from build123d import *

# Parameters (mm, degrees)
BOSS_EXTRUDE1_DEPTH = 25
SKETCH2_R           = 1.75
CUT_EXTRUDE1_DEPTH  = 40.67366885


with BuildPart() as part:
    # Sketch1 → Boss-Extrude1 (new, symmetric)
    with BuildSketch(Plane(origin=(0, 0, 0), x_dir=(0, 0, -1), z_dir=(1, 0, 0))):
        with BuildLine():
            Line((-10, 15), (-10, 0))
            Line((-10, 0), (-18, 0))
            Line((-18, 0), (-18, 1.5))
            Line((-18, 1.5), (-11.5, 1.5))
            Line((-11.5, 1.5), (-11.5, 15))
            ThreePointArc((-11.5, 15), (0, 26.5), (11.5, 15))
            Line((11.5, 15), (11.5, 1.5))
            Line((11.5, 1.5), (18, 1.5))
            Line((18, 1.5), (18, 0))
            Line((18, 0), (10, 0))
            Line((10, 0), (10, 15))
            ThreePointArc((10, 15), (0, 25), (-10, 15))
        make_face()
    extrude(amount=BOSS_EXTRUDE1_DEPTH, both=True)

    # Sketch2 → Cut-Extrude1 (cut, through all)
    with BuildSketch(Plane(origin=(0, 1.5, 0), x_dir=(1, 0, 0), z_dir=(0, 1, 0))):
        with Locations(Location((-15, 14.75, 0), (0, 0, 270))):
            Circle(SKETCH2_R)
        with Locations(Location((-15, -14.75, 0), (0, 0, 270))):
            Circle(SKETCH2_R)
    cut_extrude1 = extrude(amount=-CUT_EXTRUDE1_DEPTH, mode=Mode.SUBTRACT)

    # Mirror1: Cut-Extrude1 across plane
    add(cut_extrude1.mirror(Plane(origin=(0, 0, 0), x_dir=(0, 0, 1), z_dir=(1, 0, 0))), mode=Mode.SUBTRACT)


solid = part.part
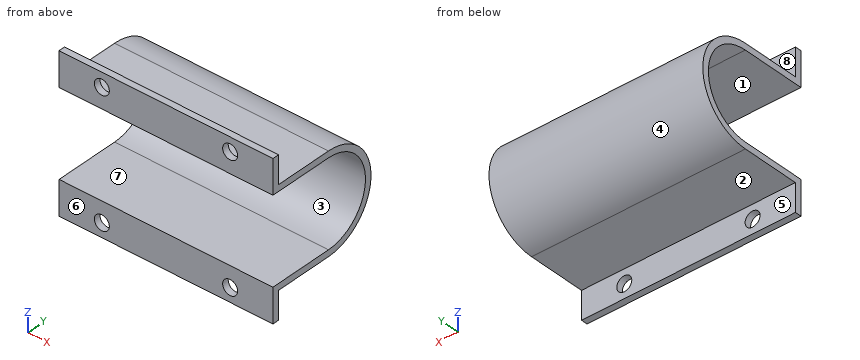
For this review, take the finished solid that the model builds, in its own axes (mm). Face numbers are marked on the shaded views. A direction names the side the tool comes from. Round coordinates to 2 decimals unless told otherwise and drop trailing zeros. Write each loop counter-clockwise with the first axis right and the second up, starting at its lowest first coordinate (ties: lowest second). Pieces come first, ordered by that corner, then holes. Notation, with made-up numbers: M 58.25,80.25 L 105.25,80.25 A9 cw 105.25,88.25 Z; hole C 76,63.25 d10. An arc over 180 degrees is marked long. Write item = value, one per line. Start each with the question number.
(1) For the marked faces 5, 6, 7 and 8, list the 3-axis set-ups (+Z, -Z, +X, -X, +Y, -Y) from which the entire face can be reached by the end or side of a thin tool; tool diameter is ignored.
(2) We need section B-B (x = 15). Give the boundary of the cut face in (y, z), then the cut area to 3 significant figures.
(3) Clearance check with flat-ended pins moving along their axes: pin 1 Ø10 at (x, y) = (18, 11) entering from +Z; pin 2 Ø6 at (x, y) = (11.5, 8.5) entering from -Z; pin 3 Ø10 at (x, y) = (-2.5, 22) entering from -Z; pin 4 Ø2 at (x, z) = (15, -14.75) entering from -Y. State where each tip first meets the part, or that it passes through.
(4) We need section C-C (y = 7.5). Give the boundary of the cut face in (x, z), then the cut area to 3 significant figures.
(5) The part is to be moulded in two halves that separate along Z. For the marked faces 1, 2, 3 and 4, say which applies: +Z half, -Z half, draft (parallel to the pull), parting line (faces both ways), or undercut.
(6) For line 1 along Z through (x, y) = (15, 0.6); line 2 along X through (y, z) = (0.8, -14.75); line 3 along Z through (x, y) = (22, 12), list the stretches that pass through material, from the lowest coordinate up.
(7) We need section A-A (z = 14.75). Give the boundary of the cut face in (x, y), then the cut area to 3 significant figures.
(8) We need section D-D (x = 20.5). Give the boundary of the cut face in (y, z).
Results found:
q1.face_5 = -Z, +X, -X, +Y
q1.face_6 = +Z, -Z, +X, -X, -Y
q1.face_7 = +X, -X, -Y
q1.face_8 = +Z, +X, -X, +Y
q2.outline = M 0,-18 L 1.5,-18 L 1.5,-16.5 L 0,-16.5 Z; M 0,-13 L 1.5,-13 L 1.5,-11.5 L 15,-11.5 A11.5 ccw 15,11.5 L 1.5,11.5 L 1.5,13 L 0,13 L 0,10 L 15,10 A10 cw 15,-10 L 0,-10 Z; M 0,16.5 L 1.5,16.5 L 1.5,18 L 0,18 Z
q2.area = 105 mm²
q3.pin_1 = 11.5
q3.pin_2 = -11.5
q3.pin_3 = -11.32
q3.pin_4 = through
q4.outline = M -25,-11.5 L 25,-11.5 L 25,-10 L -25,-10 Z; M -25,10 L 25,10 L 25,11.5 L -25,11.5 Z
q4.area = 150 mm²
q5.face_1 = undercut
q5.face_2 = -Z half
q5.face_3 = undercut
q5.face_4 = parting line
q6.line_1 = -18 to -16.5, -13 to -10, 10 to 13, 16.5 to 18
q6.line_2 = -25 to -16.75, -13.25 to 13.25, 16.75 to 25
q6.line_3 = -11.5 to -10, 10 to 11.5
q7.outline = M -25,0 L -16.75,0 L -16.75,1.5 L -25,1.5 Z; M -13.25,0 L 13.25,0 L 13.25,1.5 L -13.25,1.5 Z; M 16.75,0 L 25,0 L 25,1.5 L 16.75,1.5 Z
q7.area = 64.5 mm²
q8.outline = M 0,-18 L 1.5,-18 L 1.5,-11.5 L 15,-11.5 A11.5 ccw 15,11.5 L 1.5,11.5 L 1.5,18 L 0,18 L 0,10 L 15,10 A10 cw 15,-10 L 0,-10 Z
